For this review, use the dimensioned drawing (mm, ordinates from the lowest corner) and the shaded views. A direction names the side the tool comes from. Round coordinates to 2 decimals unless told otherwise and drop trailing zeros. Loops run counter-clockwise (first coordinate to the right, second up) from the corner with the lowest first, then second, coordinate; pieces in that order, holes last. Notation, with made-up numbers: (58, 51) -> (67, 51) arc R30 cw to (67, 85) -> close; hole circle Ø5 at (40.25, -15). An arc over 180 degrees is marked (long way). Write each question's results on one line, items separated by ' | '. Start each with the question number.
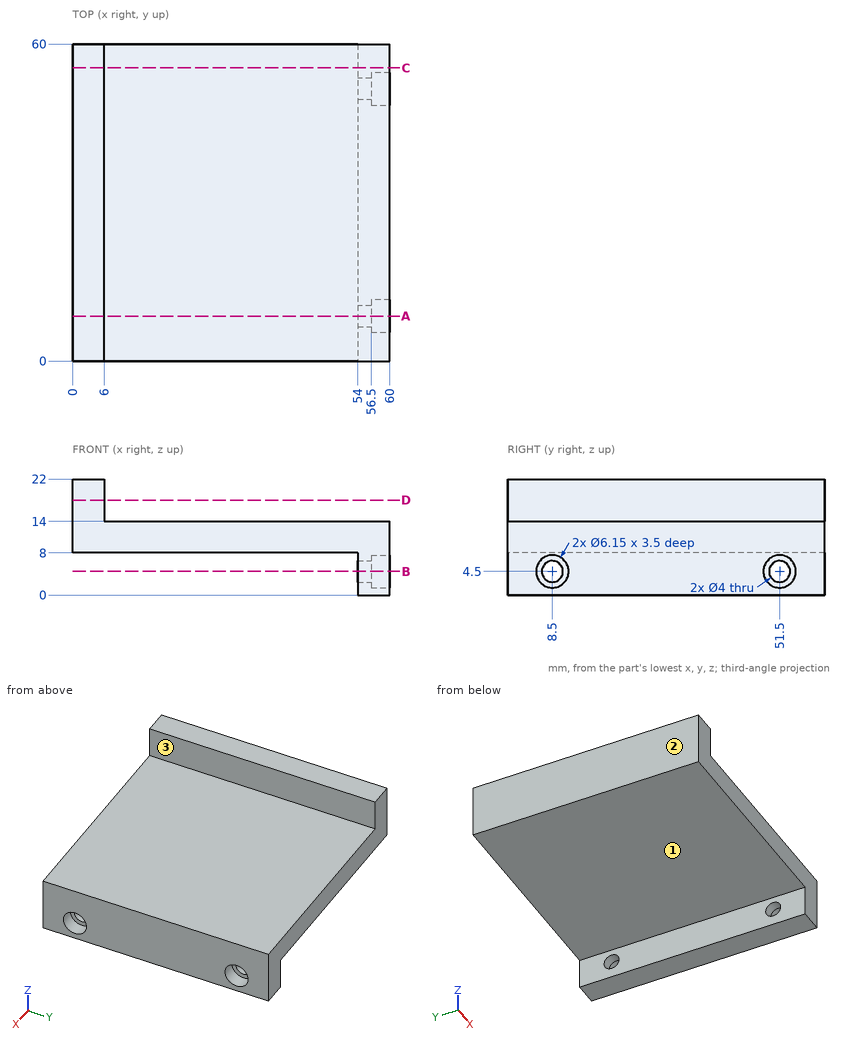
1) Take a section at D-D (z = 18). Write out the cut boundary in (x, y), plus the area to 3 significant figures.
2) Insertion check: pin 1 (1.5 mm diameter, centred on x = 19, y = 44.5, fed in from +Z); pin 2 (6.5 mm diameter, centred on y = 51.5, z = 4.5, fed in from -X); pin 3 (3.5 mm diameter, centred on y = 8.5, z = 4.5, fed in from -X); pin 4 (2 mm diameter, centred on x = 20.5, y = 34, fed in from -Z). Each pin has a flat end and moves straight along its axis. Give the tip position at first contact, or say it passes through.
3) Take a section at B-B (z = 4.5). Write out the cut boundary in (x, y) (3 decimals), plus the area to 3 significant figures.
4) Take a section at A-A (y = 8.5). Write out the cut boundary in (x, z) (3 decimals), plus the area to 3 significant figures.
5) Take a section at C-C (y = 55.5). Write out the cut boundary in (x, z), plus the area to 3 significant figures.
6) For the marked faces 1, 2 and 3, list the 3-axis set-ups (+Z, -Z, +X, -X, +Y, -Y) from which the entire face can be reached by the end or side of a thin tool; tool diameter is ignored.
7) To check wall thickness, follow line 1 (Z direction, x = 54.6, y = 8.5); line 2 (Z direction, x = 58.7, y = 8.5) (3 decimals); line 3 (X direction, y = 15, z = 17). State the ranges of each line that lie inside material, in increasing order. Write a range as from..to.
Geometry check:
1) outline: (0, 0) -> (6, 0) -> (6, 60) -> (0, 60) -> close | area: 360 mm^2
2) pin 1: stops at z = 14 | pin 2: stops at x = 54 | pin 3: passes through | pin 4: stops at z = 8
3) outline: (54, 0) -> (60, 0) -> (60, 5.425) -> (56.5, 5.425) -> (56.5, 6.5) -> (54, 6.5) -> close; (54, 10.5) -> (56.5, 10.5) -> (56.5, 11.575) -> (60, 11.575) -> (60, 48.425) -> (56.5, 48.425) -> (56.5, 49.5) -> (54, 49.5) -> close; (54, 53.5) -> (56.5, 53.5) -> (56.5, 54.575) -> (60, 54.575) -> (60, 60) -> (54, 60) -> close | area: 297 mm^2
4) outline: (0, 8) -> (54, 8) -> (54, 6.5) -> (56.5, 6.5) -> (56.5, 7.575) -> (60, 7.575) -> (60, 14) -> (6, 14) -> (6, 22) -> (0, 22) -> close; (54, 0) -> (60, 0) -> (60, 1.425) -> (56.5, 1.425) -> (56.5, 2.5) -> (54, 2.5) -> close | area: 424 mm^2
5) outline: (0, 8) -> (54, 8) -> (54, 0) -> (60, 0) -> (60, 14) -> (6, 14) -> (6, 22) -> (0, 22) -> close | area: 456 mm^2
6) face 1: -Z, -X, +Y, -Y | face 2: +Z, -Z, -X, +Y, -Y | face 3: +Z, +X, +Y, -Y
7) line 1: z = 0..2.5, 6.5..14 | line 2: z = 0..1.425, 7.575..14 | line 3: x = 0..6
